The model under review builds one solid part; all positions refer to its coordinate system, in mm. A direction names the side the tool comes from. Round coordinates to 2 decimals unless told otherwise and drop trailing zeros. Order: outer loops, then holes, each group sorted by start corner. A loop starts at its lowest first (then second) coordinate and runs counter-clockwise, first axis right, second up. Notation, with made-up numbers: M -19,23 L 9,23 A27 cw 9,55 Z; hole C -18,-31 d8. An arc over 180 degrees is marked long. Answer as CSV lines item,"result". Start each with the question number.
from build123d import *

# Parameters (mm, degrees)
F1_DEPTH = 20
F2_DEPTH = 5
F3_R     = 1


with BuildPart() as f1:
    # F0 (on Top) → F1 (new body)
    with BuildSketch(Plane.XY):
        with BuildLine():
            ThreePointArc((-16.3095064303, -2.5), (-1.253623528, 16.4523076816), (16.5, 0))
            ThreePointArc((16.5, 0), (16.4523076816, -1.253623528), (16.3095064303, -2.5))
            Line((16.3095064303, -2.5), (18.3303027798, -2.5))
            ThreePointArc((18.3303027798, -2.5), (18.4575269393, -1.2528764052), (18.5, 0))
            ThreePointArc((18.5, 0), (-1.2528764052, 18.4575269393), (-18.3303027798, -2.5))
            Line((-18.3303027798, -2.5), (-16.3095064303, -2.5))
        make_face()
        with BuildLine():
            Line((18.3303027798, -2.5), (16.3095064303, -2.5))
            ThreePointArc((16.3095064303, -2.5), (15.7866929949, -4.7989920072), (14.9415527975, -7))
            Line((14.9415527975, -7), (17.1245437895, -7))
            ThreePointArc((17.1245437895, -7), (17.8696400723, -4.7881064823), (18.3303027798, -2.5))
        make_face()
        with BuildLine():
            ThreePointArc((-14.9415527975, -7), (-15.7866929949, -4.7989920072), (-16.3095064303, -2.5))
            Line((-16.3095064303, -2.5), (-18.3303027798, -2.5))
            ThreePointArc((-18.3303027798, -2.5), (-17.8696400723, -4.7881064823), (-17.1245437895, -7))
            Line((-17.1245437895, -7), (-14.9415527975, -7))
        make_face()
    extrude(amount=F1_DEPTH)

    # F0 (on Top) → F2 (cut)
    with BuildSketch(Plane.XY):
        with BuildLine():
            ThreePointArc((-14.9415527975, -7), (-15.7866929949, -4.7989920072), (-16.3095064303, -2.5))
            Line((-16.3095064303, -2.5), (-18.3303027798, -2.5))
            ThreePointArc((-18.3303027798, -2.5), (-17.8696400723, -4.7881064823), (-17.1245437895, -7))
            Line((-17.1245437895, -7), (-14.9415527975, -7))
        make_face()
        with BuildLine():
            Line((18.3303027798, -2.5), (16.3095064303, -2.5))
            ThreePointArc((16.3095064303, -2.5), (15.7866929949, -4.7989920072), (14.9415527975, -7))
            Line((14.9415527975, -7), (17.1245437895, -7))
            ThreePointArc((17.1245437895, -7), (17.8696400723, -4.7881064823), (18.3303027798, -2.5))
        make_face()
    extrude(amount=F2_DEPTH, mode=Mode.SUBTRACT)

    # F3
    f3_edges = [f1.edges().sort_by_distance(p)[0] for p in [
        (0, 18.5, 20),
        (0, 18.5, 0),
    ]]
    fillet(f3_edges, radius=F3_R)


solid = f1.part
Item 1: For pin 1 (0.6 mm diameter, centred on x = -17.5, z = 3.5, fed in from -Y); pin 2 (3 mm diameter, centred on x = 2.5, z = 7.5, fed in from +Y); pin 3 (6 mm diameter, centred on x = 8, z = 14, fed in from -Y), all flat-tipped, find the tip position at first contact; note any pin that passes through.
Item 2: Consider section A-A (z = 8). State the section outline as (x, y) points, and give its area (3 significant figures).
Item 3: Tool access review of faces 1 (the flat face through (17, -5, 5)), 2 (the flat face through (-4, 16.2, 20)): name each direction out of +Z, -Z, +X, -X, +Y, -Y from which nothing blocks a thin tool from reaching the whole face with its end or side.
Item 4: Wall thickness on probe 1 along Y at (x, z) = (-0.5, 15); probe 2 along X at (y, z) = (0, 4); probe 3 along X at (y, z) = (6, 6): over which ranges is each line inside the solid? List them lowest first. Write a range as [from, to].
Reported:
1,pin 1,"stops at y = -2.5"
1,pin 2,"stops at y = 18.47"
1,pin 3,"stops at y = 12.3"
2,outline,"M -17.12,-7 L -14.94,-7 A16.5 cw long 14.94,-7 L 17.12,-7 A18.5 ccw long Z"
2,area,"139 mm²"
3,face 1,"-Z, +X, -X, -Y"
3,face 2,"+Z, +X, -X, +Y, -Y"
4,probe 1,"y = [16.49, 18.49]"
4,probe 2,"x = [-18.5, -16.5], [16.5, 18.5]"
4,probe 3,"x = [-17.5, -15.37], [15.37, 17.5]"
